Read the model definition and answer for the solid it produces. Units are mm, in the model's axes. Coordinates: 2 decimals unless noted, no trailing zeros. Order: outer loops, then holes, each group sorted by start corner. A loop starts at its lowest first (then second) coordinate and runs counter-clockwise, first axis right, second up. Notation, with made-up numbers: M 64,-18 L 86,-18 A24 cw 86,17 Z; hole C 57,24.5 d6. An arc over 180 degrees is marked long. Write each question's results on one line, items separated by ' | '.
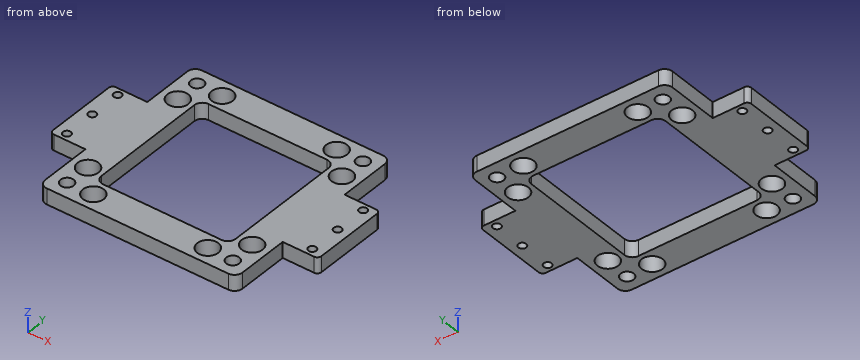
Autodesk Inventor part; units mm, degrees
ref_plane "Work Plane1" through (-32.5, -32.5, -1) normal (0, 0, -1) x (0, 1, 0)
ref_plane "YZ Plane" through (0, 0, 0) normal (1, 0, 0) x (0, 1, 0)
ref_plane "XZ Plane" through (0, 0, 0) normal (0, 1, 0) x (-1, 0, 0)
sketch "Sketch1" plane through (0, 0, 0) normal (0, 0, 1) x (1, 0, 0)
  line L0 (-25, 25) -> (25, 25)
  line L1 (25, 25) -> (25, -25)
  line L2 (25, -25) -> (-25, -25)
  line L3 (-25, -25) -> (-25, 25)
  line L4 (-25, 25) -> (25, -25) construction
  line L5 (25, 25) -> (-25, -25) construction
  circle A0 centre (0, 0) radius 2.5
  circle A1 centre (-20.8, -14.5) radius 2.65
  circle A2 centre (-14.5, -20.8) radius 2.65
  circle A3 centre (-20.8, 14.5) radius 2.65
  circle A4 centre (20.8, -14.5) radius 2.65
  circle A5 centre (20.8, 14.5) radius 2.65
  circle A6 centre (-14.5, 20.8) radius 2.65
  circle A7 centre (14.5, -20.8) radius 2.65
  circle A8 centre (14.5, 20.8) radius 2.65
  dimension "d0" = 50
  dimension "d1" = 50
  dimension "d2" = 5
  dimension "d5" = 5.3
  dimension "d6" = 4.2
  dimension "d8" = 10.5
  dimension "d11" = 29
  dimension "d14" = 41.6
extrude "Extrusion1" add sketch "Sketch1" along normal blind 4
fillet "Fillet1" radius 2 4 edges at (-25, 25, 2) (25, 25, 2) (-25, -25, 2) (25, -25, 2)
sketch "Sketch2" plane through (0, 0, 4) normal (0, 0, 1) x (1, 0, 0)
  arc A0 (23, -25) -> (25, -23) centre (23, -23) ccw
  line L0 (25, -23) -> (25, 23)
  arc A1 (25, 23) -> (23, 25) centre (23, 23) ccw
  line L1 (23, 25) -> (-23, 25)
  arc A2 (-23, 25) -> (-25, 23) centre (-23, 23) ccw
  line L2 (-25, 23) -> (-25, -23)
  arc A3 (-25, -23) -> (-23, -25) centre (-23, -23) ccw
  line L3 (-23, -25) -> (23, -25)
  circle A4 centre (14.5, 20.8) radius 2.65
  circle A5 centre (-14.5, 20.8) radius 2.65
  circle A6 centre (14.5, -20.8) radius 2.65
  circle A7 centre (20.8, 14.5) radius 2.65
  circle A8 centre (20.8, -14.5) radius 2.65
  circle A9 centre (-20.8, 14.5) radius 2.65
  circle A10 centre (-14.5, -20.8) radius 2.65
  circle A11 centre (-20.8, -14.5) radius 2.65
  circle A12 centre (0, 0) radius 2.5
  line L4 (21, -21) -> (-21, -21)
  line L5 (-21, -21) -> (-21, 21)
  line L6 (-21, 21) -> (21, 21)
  line L7 (21, 21) -> (21, -21)
  line L8 (21, -21) -> (-21, 21) construction
  line L9 (-21, -21) -> (21, 21) construction
  circle A13 centre (-28.6, 21.06) radius 1.55
  dimension "d18" = 42
  dimension "d19" = 42
hole "Hole1" at (-21, 21, 4) at (21, 21, 4) at (21, -21, 4) at (-21, -21, 4) direction (0, 0, -1) diameter 3.3 end through all both
sketch "Sketch4" plane through (0, 0, 4) normal (0, 0, 1) x (1, 0, 0)
  circle A0 centre (21, -21) radius 1.65 construction
  circle A1 centre (-21, 21) radius 1.65 construction
  circle A2 centre (21, 21) radius 1.65 construction
  circle A3 centre (-21, -21) radius 1.65 construction
  arc A4 (23, -25) -> (25, -23) centre (23, -23) ccw
  line L0 (25, -23) -> (25, 23)
  arc A5 (25, 23) -> (23, 25) centre (23, 23) ccw
  line L1 (23, 25) -> (-23, 25)
  arc A6 (-23, 25) -> (-25, 23) centre (-23, 23) ccw
  line L2 (-25, 23) -> (-25, -23)
  arc A7 (-25, -23) -> (-23, -25) centre (-23, -23) ccw
  line L3 (-23, -25) -> (23, -25)
  circle A8 centre (14.5, 20.8) radius 2.65 construction
  circle A9 centre (-14.5, 20.8) radius 2.65 construction
  circle A10 centre (14.5, -20.8) radius 2.65 construction
  circle A11 centre (20.8, 14.5) radius 2.65 construction
  circle A12 centre (20.8, -14.5) radius 2.65 construction
  circle A13 centre (-20.8, 14.5) radius 2.65 construction
  circle A14 centre (-14.5, -20.8) radius 2.65 construction
  circle A15 centre (-20.8, -14.5) radius 2.65 construction
  circle A16 centre (0, 0) radius 2.5 construction
  line L4 (17, -15) -> (17, 15)
  line L5 (15, 17) -> (-15, 17)
  line L6 (-17, 15) -> (-17, -15)
  line L7 (-15, -17) -> (15, -17)
  arc A17 (15, -17) -> (17, -15) centre (15, -15) ccw
  arc A18 (-17, -15) -> (-15, -17) centre (-15, -15) ccw
  arc A19 (-15, 17) -> (-17, 15) centre (-15, 15) ccw
  arc A20 (17, 15) -> (15, 17) centre (15, 15) ccw
  dimension "d34" = 8
  dimension "d35" = 2
extrude "Extrusion2" cut sketch "Sketch4" against normal through all contours A17 L7 A18 L6 A19 L5 A20 L4
sketch "Sketch5" plane through (0, 0, 4) normal (0, 0, 1) x (1, 0, 0)
  arc A0 (17, 15) -> (15, 17) centre (15, 15) ccw construction
  line L0 (17, 15) -> (17, -15) construction
  arc A1 (15, -17) -> (17, -15) centre (15, -15) ccw construction
  line L1 (15, -17) -> (-15, -17) construction
  arc A2 (-17, -15) -> (-15, -17) centre (-15, -15) ccw construction
  line L2 (-17, -15) -> (-17, 15) construction
  arc A3 (-15, 17) -> (-17, 15) centre (-15, 15) ccw construction
  line L3 (-15, 17) -> (15, 17) construction
  circle A4 centre (21, -21) radius 1.65 construction
  circle A5 centre (-21, 21) radius 1.65 construction
  circle A6 centre (21, 21) radius 1.65 construction
  circle A7 centre (-21, -21) radius 1.65 construction
  arc A8 (23, -25) -> (25, -23) centre (23, -23) ccw construction
  line L4 (25, -23) -> (25, 23) construction
  arc A9 (25, 23) -> (23, 25) centre (23, 23) ccw construction
  line L5 (23, 25) -> (-23, 25) construction
  arc A10 (-23, 25) -> (-25, 23) centre (-23, 23) ccw construction
  line L6 (-25, 23) -> (-25, -23) construction
  arc A11 (-25, -23) -> (-23, -25) centre (-23, -23) ccw construction
  line L7 (-23, -25) -> (23, -25) construction
  circle A12 centre (14.5, 20.8) radius 2.65 construction
  circle A13 centre (-14.5, 20.8) radius 2.65 construction
  circle A14 centre (14.5, -20.8) radius 2.65 construction
  circle A15 centre (20.8, 14.5) radius 2.65 construction
  circle A16 centre (20.8, -14.5) radius 2.65 construction
  circle A17 centre (-20.8, 14.5) radius 2.65 construction
  circle A18 centre (-14.5, -20.8) radius 2.65 construction
  circle A19 centre (-20.8, -14.5) radius 2.65 construction
  circle A20 centre (31.1, -8.2) radius 1
  circle A21 centre (31.1, 0) radius 1
  circle A22 centre (31.1, 8.2) radius 1
  line L8 (25, 23) -> (25, -23)
  line L9 (33, -10) -> (25, -10)
  line L10 (25, -10) -> (25, 10)
  line L11 (25, 10) -> (33, 10)
  line L12 (0, 45.5) -> (0, -45.5) construction
  arc A23 (33, -10) -> (34, -9.0093) centre (33, -9) ccw
  arc A24 (34, 9) -> (33, 10) centre (33, 9) ccw
  line L13 (45.5, 0) -> (-45.5, 0) construction
  line L14 (-34, -9.0093) -> (-34, 9) construction
  circle A25 centre (-31.1, -8.2) radius 1
  circle A26 centre (-31.1, 0) radius 1
  circle A27 centre (-31.1, 8.2) radius 1
  line L15 (-33, -10) -> (-25, -10)
  line L16 (-25, -10) -> (-25, 10)
  line L17 (-25, 10) -> (-33, 10)
  line L18 (-34, 9) -> (-34, -9.0093)
  arc A28 (-34, -9.0093) -> (-33, -10) centre (-33, -9) ccw
  arc A29 (-33, 10) -> (-34, 9) centre (-33, 9) ccw
  line L19 (34, 9) -> (34, -9.0093)
  point P0 (0, 0)
  point P1 (34, -10)
  point P2 (32.5, 10)
  point P3 (-34, -10)
  point P4 (-32.5, 10)
  dimension "d38" = 20
  dimension "d39" = 1
  dimension "d40" = 1
  dimension "d43" = 9
ref_plane "Work Plane1" through (-32.5, -32.5, -1) normal (0, 0, -1) x (0, 1, 0)
extrude "Extrusion3" add sketch "Sketch5" against normal up to surface (4 mm away)
properties part number "20_IM_LED_holder"
(1) The part is cut by section A-A, the plane y = -8.2. Write down the section's boundary in (x, z), then the cut area to 3 significant figures.
Conclusion:
outline: M -34,0 L -32.1,0 L -32.1,4 L -34,4 Z; M -30.1,0 L -17,0 L -17,4 L -30.1,4 Z; M 17,0 L 30.1,0 L 30.1,4 L 17,4 Z; M 32.1,0 L 34,0 L 34,4 L 32.1,4 Z | area: 120 mm²
(2) Given pin 1 (1.8 mm diameter, centred on x = -31.1, y = 8.2, fed in from -Z); pin 2 (2 mm diameter, centred on x = -28.5, z = 1.5, fed in from -Y); pin 3 (1.2 mm diameter, centred on y = -18.5, z = 2.5, fed in from -X), each flat-ended and moving along its own axis, determine where each tip first touches the part or whether it passes through.
Conclusion:
pin 1: through | pin 2: y = -10 | pin 3: x = -25
(3) The part is cut by section D-D, the plane y = 20.8. Write down the section's boundary in (x, z), then the cut area to 3 significant figures.
Conclusion:
outline: M -25,0 L -22.64,0 L -22.64,4 L -25,4 Z; M -19.36,0 L -17.15,0 L -17.15,4 L -19.36,4 Z; M -11.85,0 L 11.85,0 L 11.85,4 L -11.85,4 Z; M 17.15,0 L 19.36,0 L 19.36,4 L 17.15,4 Z; M 22.64,0 L 25,0 L 25,4 L 22.64,4 Z | area: 131 mm²
(4) Straight lines are drawn through the part: line 1 (Y direction, x = -20.8, z = 3.25); line 2 (Y direction, x = 14.5, z = 2.5); line 3 (X direction, y = 21, z = 2.15). For each, find the intervals that lie inside material, in ascending order.
Conclusion:
line 1: -25 to -22.64, -19.36 to -17.15, -11.85 to 11.85, 17.15 to 19.36, 22.64 to 25 | line 2: -25 to -23.45, -18.15 to -17, 17 to 18.15, 23.45 to 25 | line 3: -25 to -22.65, -19.35 to -17.14, -11.86 to 11.86, 17.14 to 19.35, 22.65 to 25
(5) The part is cut by section B-B, the plane x = -31.1. Write down the section's boundary in (y, z), then the cut area to 3 significant figures.
Conclusion:
outline: M -10,0 L -9.2,0 L -9.2,4 L -10,4 Z; M -7.2,0 L -1,0 L -1,4 L -7.2,4 Z; M 1,0 L 7.2,0 L 7.2,4 L 1,4 Z; M 9.2,0 L 10,0 L 10,4 L 9.2,4 Z | area: 56.0 mm²
(6) The part is cut by section C-C, the plane x = -21. Write down the section's boundary in (y, z).
Conclusion:
outline: M -25,0 L -22.65,0 L -22.65,4 L -25,4 Z; M -19.35,0 L -17.14,0 L -17.14,4 L -19.35,4 Z; M -11.86,0 L 11.86,0 L 11.86,4 L -11.86,4 Z; M 17.14,0 L 19.35,0 L 19.35,4 L 17.14,4 Z; M 22.65,0 L 25,0 L 25,4 L 22.65,4 Z
